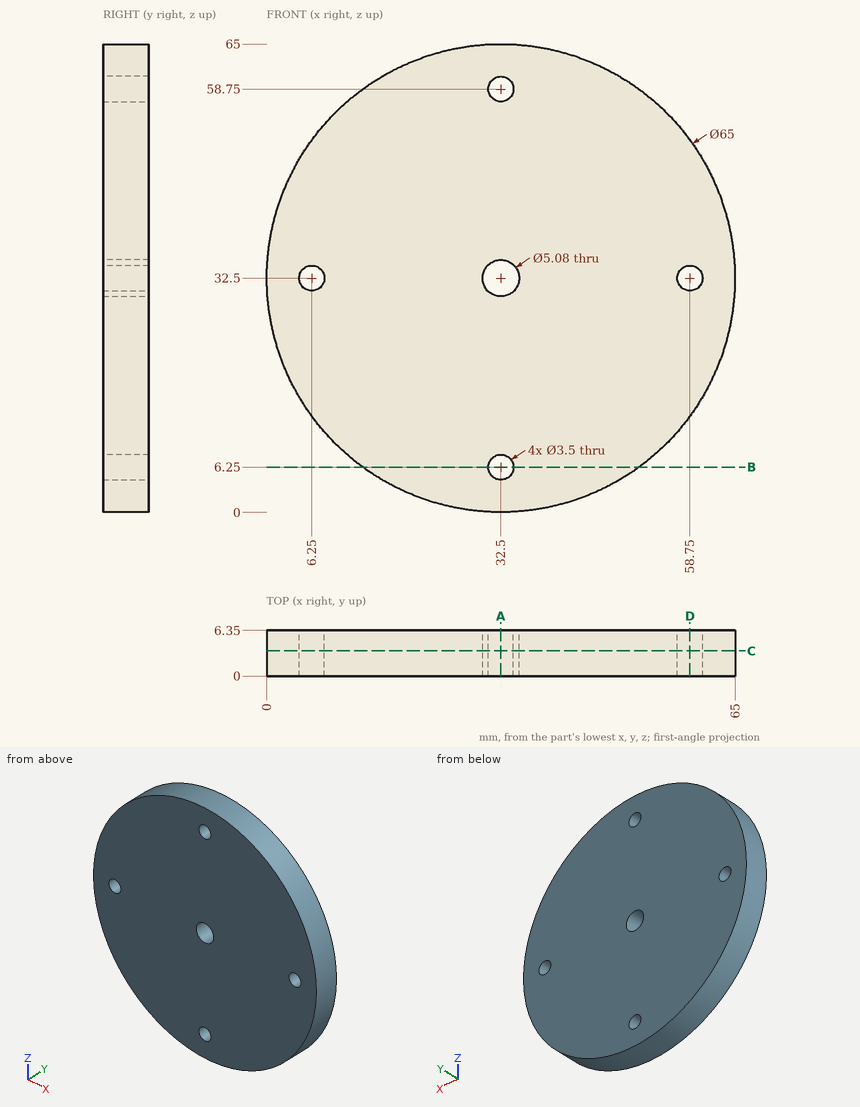
The figure shows three views and two pictorial views of one solid part (mm, origin at its lowest corner). Answer the questions. Give positions to 0.01 mm unless a question says otherwise; leave off trailing zeros. Write each loop counter-clockwise with the first axis right and the second up, starting at its lowest first coordinate (ties: lowest second). Pieces come first, ordered by that corner, then holes. Notation, with made-up numbers: (4.5, 67) - (41.5, 67) arc R11 ccw to (41.5, 83) - close; hole circle Ø11 at (43.25, -27). An arc over 180 degrees is marked (long way). Return JSON: item names as keys, results as strings.
Q1. Consider line 1 along X through (y, z) = (3.75, 32.5); line 2 along Z through (x, y) = (33, 0.5); line 3 along X through (y, z) = (3.25, 58.75). Determine where each line is inside the solid, lowest interval first. Write a range as [from, to].
Reply:
{"line 1": "[0, 4.5], [8, 29.96], [35.04, 57], [60.5, 65]", "line 2": "[0, 4.57], [7.93, 30.01], [34.99, 57.07], [60.43, 65]", "line 3": "[13.34, 30.75], [34.25, 51.66]"}
Q2. A cutting plane is placed at A-A, the plane x = 32.5. Determine the outline of the cut face in (y, z), and give its area (3 significant figures).
Reply:
{"outline": "(0, 0) - (6.35, 0) - (6.35, 4.5) - (0, 4.5) - close; (0, 8) - (6.35, 8) - (6.35, 29.96) - (0, 29.96) - close; (0, 35.04) - (6.35, 35.04) - (6.35, 57) - (0, 57) - close; (0, 60.5) - (6.35, 60.5) - (6.35, 65) - (0, 65) - close", "area": "336 mm²"}
Q3. Given P1, Ø2, axis at x = 32.5, z = 6.25, coming from the -Y side, flat-ended and moving along its own axis, determine where the tip first touches the part or whether it passes through.
Reply:
{"P1": "through"}
Q4. A cutting plane is placed at B-B, the plane z = 6.25. Determine the outline of the cut face in (x, y).
Reply:
{"outline": "(13.34, 0) - (30.75, 0) - (30.75, 6.35) - (13.34, 6.35) - close; (34.25, 0) - (51.66, 0) - (51.66, 6.35) - (34.25, 6.35) - close"}
Q5. A cutting plane is placed at D-D, the plane x = 58.75. Determine the outline of the cut face in (y, z), and give its area (3 significant figures).
Reply:
{"outline": "(0, 13.34) - (6.35, 13.34) - (6.35, 30.75) - (0, 30.75) - close; (0, 34.25) - (6.35, 34.25) - (6.35, 51.66) - (0, 51.66) - close", "area": "221 mm²"}
Q6. A cutting plane is placed at C-C, the plane y = 3.5. Determine the outline of the cut face in (x, z).
Reply:
{"outline": "circle Ø65 at (32.5, 32.5); hole circle Ø3.5 at (6.25, 32.5); hole circle Ø5.08 at (32.5, 32.5); hole circle Ø3.5 at (32.5, 6.25); hole circle Ø3.5 at (32.5, 58.75); hole circle Ø3.5 at (58.75, 32.5)"}
